Verification items for this drawing (mm, ordinates from the low corner). A direction names the side the tool comes from. Round coordinates to 2 decimals unless told otherwise and drop trailing zeros. Order: outer loops, then holes, each group sorted by start corner. A loop starts at its lowest first (then second) coordinate and runs counter-clockwise, first axis right, second up. Notation, with made-up numbers: (-31, -25) -> (-13, -25) arc R21 ccw to (-13, -6) -> close; hole circle Ø11 at (-3, 29). An arc over 180 degrees is marked (long way). Return JSON: item names as keys, results as strings. Group by question number.
Item 1: Sectioned sample at B-B on x = 38. Record the cut outline in (y, z), plus the area to 4 significant figures.
Item 2: Access from +Z, -Z, +X, -X, +Y, -Y to the whole of each face (thin tool, end or side, straight path). Record for the marked faces 1, 2 and 3.
Item 3: Sectioned sample at D-D on y = 38.5. Record the cut outline in (x, z), plus the area to 3 significant figures.
Item 4: Draft check along X on the marked faces 4, 5, 6 and 7. Enter one of: pulls with the +X half, pulls with the -X half, needs draft (parallel to the pull), parting line crosses it, or undercut.
Item 5: Depth check by flat-ended pin: pin 1 Ø4 at (x, y) = (30, 43.5) entering from +Z; pin 2 Ø5 at (x, z) = (57.5, 22) entering from -Y; pin 3 Ø8.5 at (x, z) = (48, 41.5) entering from -Y. Enter the tip coordinate at first touch or a pass-through.
Item 6: Scan lines: probe 1 along Y at (x, z) = (26, 45); probe 2 along Y at (x, z) = (59, 16.5); probe 3 along Z at (x, y) = (80.5, 53.5) (1 decimal). Record each from-to range of solid material in increasing order. Write a range as from..to.
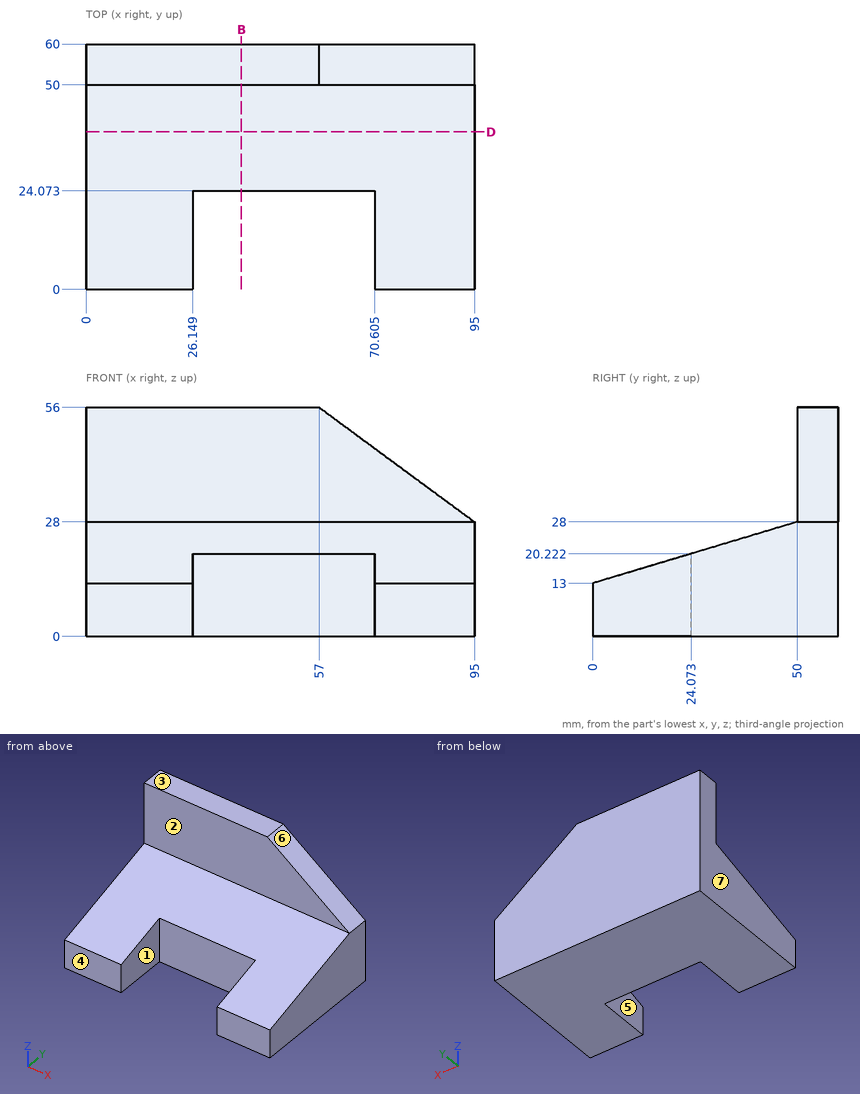
Recorded:
{
 "1": {"outline": "(24.07, 0) -> (60, 0) -> (60, 56) -> (50, 56) -> (50, 28) -> (24.07, 20.22) -> close", "area": "1,185 mm²"},
 "2": {"face 1": "+Z, -Z, -Y", "face 2": "+Z, +X, -X, -Y", "face 3": "+Z, +X, -X, +Y, -Y"},
 "3": {"outline": "(0, 0) -> (95, 0) -> (95, 24.55) -> (0, 24.55) -> close", "area": "2,330 mm²"},
 "4": {"face 4": "needs draft", "face 5": "undercut", "face 6": "pulls with the +X half", "face 7": "pulls with the -X half"},
 "5": {"pin 1": "z = 26.65", "pin 2": "y = 24.07", "pin 3": "y = 50"},
 "6": {"probe 1": "50..60", "probe 2": "24.07..60", "probe 3": "0..38.7"}
}
